Model file for the job. Use its own axes, mm. A direction names the side the tool comes from. Round coordinates to 2 decimals unless told otherwise and drop trailing zeros. Write each loop counter-clockwise with the first axis right and the second up, starting at its lowest first coordinate (ties: lowest second). Pieces come first, ordered by that corner, then holes.
```python
from build123d import *

# Parameters (mm, degrees)
F0_W     = 20
F0_H     = 2.5
F1_DEPTH = 36
F5_W     = 108.4840968251
F5_H     = 66.9420473278
F6_DEPTH = 25


with BuildPart() as f1:
    # F0 (on Top) → F1 (new body)
    with BuildSketch(Plane.XY):
        Polygon((-11.042611652, 7.0852233041), (-10, 5), (0, 10), (0, 12.5), align=None)
        Polygon((0, 0), (-20, 0), (-10, 5), (-11.042611652, 7.0852233041), (-30.5902134255, -2.5), (0, -2.5), align=None)
        Polygon((20, 0), (0, 0), (0, -2.5), (64.9998660191, -2.5), (20, 12.5), (20, 10), (50, 0), align=None)
        with Locations((10, 11.25)):
            Rectangle(F0_W, F0_H)
    extrude(amount=F1_DEPTH)

    # F3: sweep along a path in F2
    with BuildLine(Plane.YZ) as f3_path:
        Line((12.28813377, 36), (-2.71186623, 46))
    # F1_face (on face) → F3 (sweep)
    with BuildSketch(Plane(origin=(15.9254159415, 2.5999378956, 36), x_dir=(1, 0, 0), z_dir=(0, 0, 1))):
        Polygon((-15.9254159415, 9.9000621044), (-46.515629367, -5.0999378956), (49.0744500776, -5.0999378956), (4.0745840585, 9.9000621044), align=None)
        Polygon((4.0745840585, 7.4000621044), (34.0745840585, -2.5999378956), (-35.9254159415, -2.5999378956), (-15.9254159415, 7.4000621044), align=None, mode=Mode.SUBTRACT)
    sweep(path=f3_path.line)

    # F4: sweep along a path in F2
    with BuildLine(Plane.YZ) as f4_path:
        Line((12.28813377, 0), (-2.71186623, -10))
    # F1_face1 (on face) → F4 (sweep)
    with BuildSketch(Plane(origin=(15.9254159415, 2.5999378956, 0), x_dir=(1, 0, 0), z_dir=(0, 0, -1))):
        Polygon((-46.515629367, 5.0999378956), (-15.9254159415, -9.9000621044), (4.0745840585, -9.9000621044), (49.0744500776, 5.0999378956), align=None)
        Polygon((34.0745840585, 2.5999378956), (4.0745840585, -7.4000621044), (-15.9254159415, -7.4000621044), (-35.9254159415, 2.5999378956), align=None, mode=Mode.SUBTRACT)
    sweep(path=f4_path.line)

    # F5 (on Front) → F6 (cut)
    with BuildSketch(Plane.XZ):
        with Locations((17.6961012185, 16.9055629522)):
            Rectangle(F5_W, F5_H)
    extrude(amount=F6_DEPTH, mode=Mode.SUBTRACT)


solid = f1.part
```
1) Cut at C-C on y = 4.25. List the corners of the cut face in (x, z).
2) Cut at A-A on z = 33.5. List the corners of the cut face in (x, y), and give its area (3 significant figures).
3) Which spindle directions (+Z, -Z, +X, -X, +Y, -Y) get a long thin tool onto all of the face, cutting with end or side? Do faces 5 (the face through (-8.33, 4.86, 38.37)), 6 (the face through (30.6, 3.62, 37.9)). Say none if no direction does.
4) Wall check: probe 1 along Y at (x, z) = (12.5, 13); probe 2 along Z at (x, y) = (22.5, 6.75); probe 3 along Z at (x, y) = (-5.5, 6). Give the ranges that are in metal, low to high.
5) Pull direction Z, two halves, no side cores. Call faces 1 (the face through (31.02, 3.48, -1.9)), 2 (the face through (10, 10, 18)), 3 (the face through (33.8, 4.3, 38.4)), 4 (the face through (-8.14, 3.56, -3.3)): released by +Z, released by -Z, zero draft, split by the parting line, or undercut.
6) Cut at B-B on x = 10. List the corners of the cut face in (y, z).
7) Cut at D-D on x = 29.5. List the corners of the cut face in (y, z), and give its area (3 significant figures).
8) Flat gauge pins, fed straight in: pin 1 Ø2 at (x, y) = (-5, 3) entering from -Z; pin 2 Ø5 at (x, y) = (30.5, 8) entering from +Z; pin 3 Ø6 at (y, z) = (5.5, 10.5) entering from -X; pin 4 Ø2 at (x, y) = (-9, 9.5) entering from -Z. Where does each tip first touch, or does it go through?
Result sheet:
1. outline: (-16.82, 0) - (0, -5.5) - (20, -5.5) - (44.75, 0) - (44.75, 36) - (20, 41.5) - (0, 41.5) - (-16.82, 36) - close; hole (-11.5, 0) - (0, -3.83) - (20, -3.83) - (37.25, 0) - (37.25, 36) - (20, 39.83) - (0, 39.83) - (-11.5, 36) - close
2. outline: (-25.49, 0) - (-20, 0) - (0, 10) - (20, 10) - (50, 0) - (57.5, 0) - (20, 12.5) - (0, 12.5) - close
2. area: 194 mm2
3. face 5: +Z, -X, +Y
3. face 6: -Y
4. probe 1: y = 10 to 12.5
4. probe 2: z = -3.28 to -1.61, 37.61 to 39.28
4. probe 3: z = -2.54 to -0.83, 36.83 to 38.54
5. face 1: undercut
5. face 2: undercut
5. face 3: released by +Z
5. face 4: released by -Z
6. outline: (0, -8.33) - (12.5, 0) - (12.5, 36) - (0, 44.33) - (0, 42.67) - (10, 36) - (10, 0) - (0, -6.67) - close
7. outline: (0, -6.22) - (9.33, 0) - (9.33, 36) - (0, 42.22) - (0, 40.56) - (6.83, 36) - (6.83, 0) - (0, -4.56) - close
7. area: 117 mm2
8. pin 1: stops at z = -5.44
8. pin 2: stops at z = 38.42
8. pin 3: stops at x = -20.39
8. pin 4: passes through
